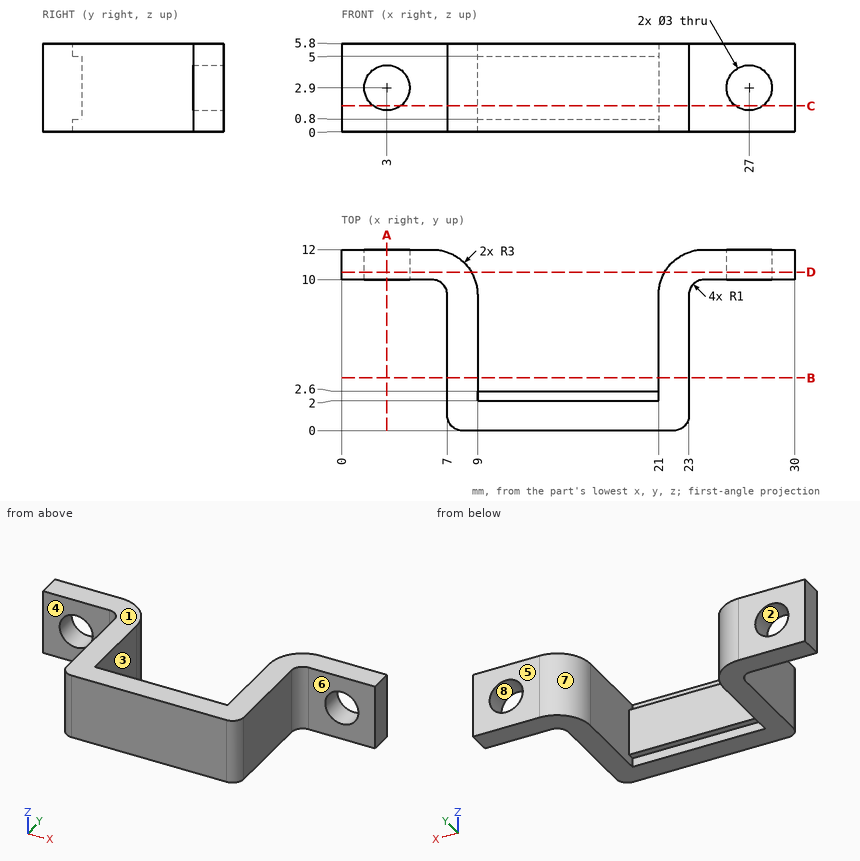
Study the drawing (mm; zero at the part's minimum x, y, z) and answer. A direction names the side the tool comes from. Give positions to 0.01 mm unless a question says otherwise; leave off trailing zeros. Write each loop counter-clockwise with the first axis right and the second up, starting at its lowest first coordinate (ties: lowest second). Pieces come first, ordered by that corner, then holes. Notation, with made-up numbers: (45, -20.5) - (98, -20.5) arc R11 ccw to (98, -9.5) - close; hole circle Ø1 at (22, -27). An arc over 180 degrees is marked (long way). Write item = value, one per line. Start each with the question number.
Item 1: Find section C-C (z = 1.7). Give the vertices of the cut face in (x, y).
Item 2: Find section D-D (y = 10.5). Give the vertices of the cut face in (x, z), then the cut area to 3 significant figures.
Item 3: Find section B-B (y = 3.5). Give the vertices of the cut face in (x, z), then the cut area to 3 significant figures.
Item 4: Each of these flat-tipped pins is pushed along its axis until it touches: P1, Ø0.9, axis at x = 18, z = 5.5, coming from the +Y side; P2, Ø1.7, axis at y = 6.5, z = 2.5, coming from the +X side; P3, Ø0.9, axis at x = 13, z = 0.5, coming from the +Y side. Where does it stop, or does it pass through?
Item 5: Find section A-A (x = 3). Give the vertices of the cut face in (y, z), then the cut area to 3 significant figures.
Item 6: The mould has two halves that part along Z. Classify the marked faces 1, 2 and 3: +Z half, -Z half, draft (parallel to the pull), parting line (faces both ways), or undercut.
Item 7: A tool of negligible diameter and unlimited length cuts with its end or side. For the marked faces 4, 5, 6, 7 and 8, from which of +Z, -Z, +X, -X, +Y, -Y can it reach the whole face along a straight path? Write none if from no direction.
Item 8: Find the intervals of material crossed by probe 1 along X at (y, z) = (11.25, 4); probe 2 along X at (y, z) = (4.25, 3.85); probe 3 along Z at (x, y) = (3, 10.65), in increasing order. Write a range as [from, to].
Response:
q1.outline = (0, 10) - (2.1, 10) - (2.1, 12) - (0, 12) - close; (3.9, 10) - (6, 10) arc R1 cw to (7, 9) - (7, 1) arc R1 ccw to (8, 0) - (22, 0) arc R1 ccw to (23, 1) - (23, 9) arc R1 cw to (24, 10) - (26.1, 10) - (26.1, 12) - (24, 12) arc R3 ccw to (21, 9) - (21, 2.6) - (9, 2.6) - (9, 9) arc R3 ccw to (6, 12) - (3.9, 12) - close; (27.9, 10) - (30, 10) - (30, 12) - (27.9, 12) - close
q2.outline = (0, 0) - (8.6, 0) - (8.6, 5.8) - (0, 5.8) - close; (21.4, 0) - (30, 0) - (30, 5.8) - (21.4, 5.8) - close; hole circle Ø3 at (3, 2.9); hole circle Ø3 at (27, 2.9)
q2.area = 85.6 mm²
q3.outline = (7, 0) - (9, 0) - (9, 5.8) - (7, 5.8) - close; (21, 0) - (23, 0) - (23, 5.8) - (21, 5.8) - close
q3.area = 23.2 mm²
q4.P1 = 2
q4.P2 = 23
q4.P3 = 2.6
q5.outline = (10, 0) - (12, 0) - (12, 1.4) - (10, 1.4) - close; (10, 4.4) - (12, 4.4) - (12, 5.8) - (10, 5.8) - close
q5.area = 5.60 mm²
q6.face_1 = +Z half
q6.face_2 = undercut
q6.face_3 = draft
q7.face_4 = +Z, -Z, -X, -Y
q7.face_5 = +Z, -Z, +X, -X, +Y
q7.face_6 = +Z, -Z, +X, -Y
q7.face_7 = +Z, -Z, +Y
q7.face_8 = +Y, -Y
q8.probe_1 = [0, 1.98], [4.02, 7.98], [22.02, 25.98], [28.02, 30]
q8.probe_2 = [7, 9], [21, 23]
q8.probe_3 = [0, 1.4], [4.4, 5.8]
